Geometry check sheet. Reference: drawing and pictorial views, mm from the part's lowest x, y, z. A direction names the side the tool comes from. Round coordinates to 2 decimals unless told otherwise and drop trailing zeros. Order: outer loops, then holes, each group sorted by start corner. A loop starts at its lowest first (then second) coordinate and runs counter-clockwise, first axis right, second up. Notation, with made-up numbers: (82.5, -35.75) -> (114.5, -35.75) arc R30 cw to (114.5, 1.25) -> close; hole circle Ø1 at (41, 59.5). An arc over 180 degrees is marked (long way). Return JSON: item names as keys, results as strings. Group by question number.
1) Section check B-B on z = 21.75. Enter the section's corners in (x, y).
2) Section check A-A on y = 28. Enter the section's corners in (x, z), plus the area to 3 significant figures.
3) Scan lines: L1, parallel to Y at x = 9.75, z = 16.5; L2, parallel to Z at x = 12.5, y = 17.5; L3, parallel to Z at x = 14, y = 98. Record each from-to range of solid material in increasing order.
4) Depth check by flat-ended pin: pin 1 (5 mm diameter, centred on x = 9.5, y = 60.5, fed in from +Z); pin 2 (4 mm diameter, centred on x = 4, z = 14, fed in from +Y); pin 3 (1.5 mm diameter, centred on x = 14.5, y = 28.5, fed in from +Z); pin 4 (4 mm diameter, centred on y = 97, z = 19.5, fed in from +X). Enter the tip coordinate at first touch or a pass-through.
5) Tool access check on the marked faces 1, 2 and 3. Record the directions out of +Z, -Z, +X, -X, +Y, -Y that give a thin tool (end or side, any length) a straight path to the whole face; none if there is none.
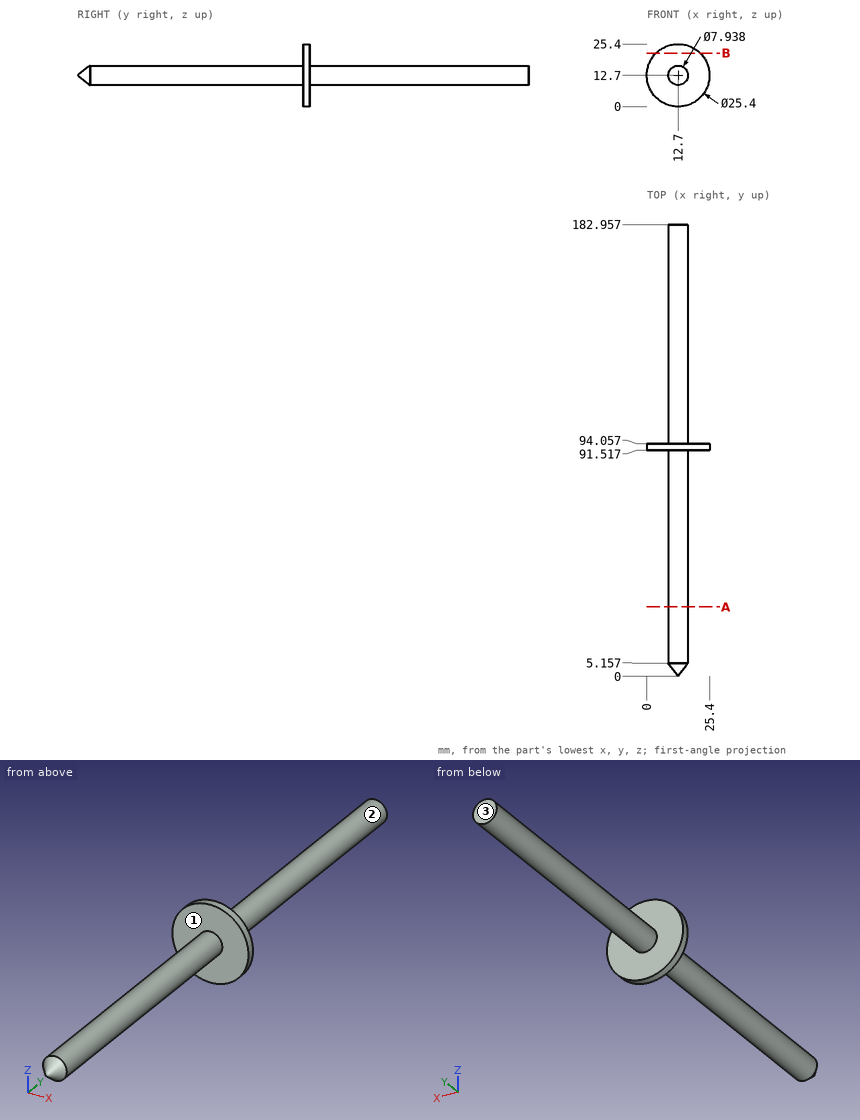
Check result:
{
 "1": {"outline": "(3.79, 91.52) -> (21.61, 91.52) -> (21.61, 94.06) -> (3.79, 94.06) -> close"},
 "2": {"outline": "circle Ø7.94 at (12.7, 12.7)", "area": "49.5 mm^2"},
 "3": {"L1": "91.52 to 94.06", "L2": "8.74 to 16.66", "L3": "8.95 to 16.45"},
 "4": {"pin 1": "z = 16.61", "pin 2": "y = 94.06", "pin 3": "z = 16.53", "pin 4": "through"},
 "5": {"face 1": "-Y", "face 2": "+Y", "face 3": "+Z, -Z, +X, -X, +Y"}
}
